CAD build for the part. Positions are in the model's coordinates, mm. A direction names the side the tool comes from. Coordinates: 2 decimals unless noted, no trailing zeros. Order: outer loops, then holes, each group sorted by start corner. A loop starts at its lowest first (then second) coordinate and runs counter-clockwise, first axis right, second up.
from build123d import *

# Parameters (mm, degrees)
F0_R      = 2.690874
F1_DEPTH  = 11
F2_W      = 4
F2_H      = 4
F1_FACE_W = 20
F1_FACE_H = 11
F3_DEPTH  = 25


with BuildPart() as f1:
    # F0 (on Front) → F1 (new body)
    with BuildSketch(Plane.XZ):
        Polygon((0, 10), (0, 0), (20, 0), (20, 20), (0, 20), align=None)
        with Locations((5.423373, 10)):
            Circle(F0_R, mode=Mode.SUBTRACT)
    extrude(amount=F1_DEPTH)

    # F2 (on Top) + F1_face (on face) → F3 (cut)
    with BuildSketch(Plane.XY):
        with Locations((18.086078, -9.081113)):
            Rectangle(F2_W, F2_H)
    with BuildSketch(Plane(origin=(10, -5.5, 20), x_dir=(1, 0, 0), z_dir=(0, 0, 1))):
        Rectangle(F1_FACE_W, F1_FACE_H)
    extrude(amount=F3_DEPTH, mode=Mode.SUBTRACT)


solid = f1.part
1) Slice it at C-C (y = -4.5). List the corners of the cut face in (x, z), plus the area to 3 significant figures.
2) Two-plate mould, pull along Z, no slides. Class faces 3 (the flat face through (10, -5, 0)), 4 (the flat face through (10, -5, 20)), 5 (the cylindrical face through (4.84, -5.423, 7.373)), 6 (the flat face through (10, -11, 10)): released by +Z, released by -Z, zero draft, split by the parting line, or undercut.
3) Slice it at D-D (z = 13.5). List the corners of the cut face in (x, y), plus the area to 3 significant figures.
4) Pin check, flat tips, straight feed: P1, Ø3, axis at x = 12.5, z = 2, coming from the +Y side; P2, Ø3, axis at x = 18, z = 8, coming from the -Y side; P3, Ø1.2, axis at y = -9.5, z = 6, coming from the +X side. Stop position of each tip, or through.
5) Which spindle directions (+Z, -Z, +X, -X, +Y, -Y) get a long thin tool onto all of the face, cutting with end or side? Do faces 1 (the flat face through (0, -5, 10)), 2 (the flat face through (16.086, -9, 10)). Say none if no direction does.
6) Slice it at B-B (x = 3). List the corners of the cut face in (y, z).
7) Slice it at A-A (z = 10). List the corners of the cut face in (x, y), plus the area to 3 significant figures.
8) Drill centre lines: probe 1 along Y at (x, z) = (18.25, 3.25); probe 2 along X at (y, z) = (-7.75, 6.75); probe 3 along X at (y, z) = (-4.75, 12). Where is each one in solid material? Low to high.
Worked out:
1. outline: (0, 0) - (20, 0) - (20, 20) - (0, 20) - close; hole circle Ø5.38 at (5.42, 10)
1. area: 377 mm2
2. face 3: released by -Z
2. face 4: released by +Z
2. face 5: undercut
2. face 6: zero draft
3. outline: (0, -11) - (16.09, -11) - (16.09, -7.08) - (20, -7.08) - (20, 0) - (0, 0) - close
3. area: 205 mm2
4. P1: stops at y = 0
4. P2: stops at y = -7.08
4. P3: stops at x = 16.09
5. face 1: +Z, -Z, -X, +Y, -Y
5. face 2: +Z, -Z, +X, -Y
6. outline: (-11, 0) - (0, 0) - (0, 8.83) - (-11, 8.83) - close; (-11, 11.17) - (0, 11.17) - (0, 20) - (-11, 20) - close
7. outline: (0, -11) - (2.73, -11) - (2.73, 0) - (0, 0) - close; (8.11, -11) - (16.09, -11) - (16.09, -7.08) - (20, -7.08) - (20, 0) - (8.11, 0) - close
7. area: 145 mm2
8. probe 1: y = -7.08 to 0
8. probe 2: x = 0 to 16.09
8. probe 3: x = 0 to 3.62, 7.22 to 20
